from build123d import *

# Parameters (mm, degrees)
SKETCH1_R           = 6
BOSS_EXTRUDE1_DEPTH = 5
SKETCH2_R           = 5.262480872
BOSS_EXTRUDE2_DEPTH = 6
SKETCH3_R           = 0.5
CUT_EXTRUDE1_DEPTH  = 6
SKETCH4_R           = 6
BOSS_EXTRUDE3_DEPTH = 0.8
SKETCH5_R           = 4.819461856
BOSS_EXTRUDE4_DEPTH = 0.4
FILLET3_R           = 0.5
SKETCH6_R           = 4
CUT_EXTRUDE2_DEPTH  = 15.860686391


with BuildPart() as part:
    # Sketch1 → Boss-Extrude1 (new body)
    with BuildSketch(Plane(origin=(0, 0, 0), x_dir=(1, 0, 0), z_dir=(0, 1, 0))):
        with Locations(Location((0, 0, 0), (0, 0, 270))):
            Circle(SKETCH1_R)
    extrude(amount=BOSS_EXTRUDE1_DEPTH)

    # Sketch2 → Boss-Extrude2 (add)
    with BuildSketch(Plane(origin=(0, 5, 0), x_dir=(1, 0, 0), z_dir=(0, 1, 0))):
        with Locations(Location((0, 0, 0), (0, 0, 270))):
            Circle(SKETCH2_R)
    extrude(amount=BOSS_EXTRUDE2_DEPTH)

    # Sketch3 → Cut-Extrude1 (cut)
    with BuildSketch(Plane(origin=(0, 11, 0), x_dir=(1, 0, 0), z_dir=(0, 1, 0))):
        with Locations((-1.603876434, 5.012113856)):
            Circle(SKETCH3_R)
        with Locations((0.023451225, 5.262428619)):
            Circle(SKETCH3_R)
        with Locations((1.648483316, 4.997620202)):
            Circle(SKETCH3_R)
        with Locations((3.112150373, 4.2436099)):
            Circle(SKETCH3_R)
        with Locations((4.271178469, 3.074205493)):
            Circle(SKETCH3_R)
        with Locations((5.012113856, 1.603876434)):
            Circle(SKETCH3_R)
        with Locations((5.262428619, -0.023451225)):
            Circle(SKETCH3_R)
        with Locations((4.997620202, -1.648483316)):
            Circle(SKETCH3_R)
        with Locations((4.2436099, -3.112150373)):
            Circle(SKETCH3_R)
        with Locations((3.074205493, -4.271178469)):
            Circle(SKETCH3_R)
        with Locations((1.603876434, -5.012113856)):
            Circle(SKETCH3_R)
        with Locations((-0.023451225, -5.262428619)):
            Circle(SKETCH3_R)
        with Locations((-1.648483316, -4.997620202)):
            Circle(SKETCH3_R)
        with Locations((-3.112150373, -4.2436099)):
            Circle(SKETCH3_R)
        with Locations((-4.271178469, -3.074205493)):
            Circle(SKETCH3_R)
        with Locations((-5.012113856, -1.603876434)):
            Circle(SKETCH3_R)
        with Locations((-5.262428619, 0.023451225)):
            Circle(SKETCH3_R)
        with Locations((-4.997620202, 1.648483316)):
            Circle(SKETCH3_R)
        with Locations((-4.2436099, 3.112150373)):
            Circle(SKETCH3_R)
        with Locations((-3.074205493, 4.271178469)):
            Circle(SKETCH3_R)
    extrude(amount=-CUT_EXTRUDE1_DEPTH, mode=Mode.SUBTRACT)

    # Sketch4 → Boss-Extrude3 (add)
    with BuildSketch(Plane(origin=(0, 11, 0), x_dir=(1, 0, 0), z_dir=(0, 1, 0))):
        with Locations(Location((0, 0, 0), (0, 0, 270))):
            Circle(SKETCH4_R)
    extrude(amount=BOSS_EXTRUDE3_DEPTH)

    # Sketch5 → Boss-Extrude4 (add)
    with BuildSketch(Plane(origin=(0, 11.8, 0), x_dir=(1, 0, 0), z_dir=(0, 1, 0))):
        with Locations(Location((0, 0, 0), (0, 0, 270))):
            Circle(SKETCH5_R)
    extrude(amount=BOSS_EXTRUDE4_DEPTH)

    # Fillet3
    # the kernel refuses this fillet: 0.5 mm, written as the material it takes off along each edge
    with BuildSketch(Plane(origin=(0, 12.2, 0), x_dir=(0, 0, 1), z_dir=(-1, 0, 0))) as fillet3_piece_1:
        with BuildLine():
            CenterArc((4.329563907, -0.5), FILLET3_R, 11.536959033, 78.463040967)
            Line((4.329563907, 0), (4.329563907, 0.01))
            Line((4.329563907, 0.01), (4.819461856, 0.01))
            Line((4.819461856, 0.01), (4.829461856, 0))
            ThreePointArc((4.829461856, 0), (4.829461856, -0.2), (4.829259815, -0.398))
            Line((4.829259815, -0.398), (4.819461856, -0.4))
        make_face()
    revolve(axis=Axis((0, 12.2, 0), (0, 1, 0)), mode=Mode.SUBTRACT)

    # Sketch6 → Cut-Extrude2 (cut, through all)
    with BuildSketch(Plane(origin=(0, 12.2, 0), x_dir=(1, 0, 0), z_dir=(0, 1, 0))):
        with Locations(Location((0, 0, 0), (0, 0, 270))):
            Circle(SKETCH6_R)
    extrude(amount=-CUT_EXTRUDE2_DEPTH, mode=Mode.SUBTRACT)


solid = part.part
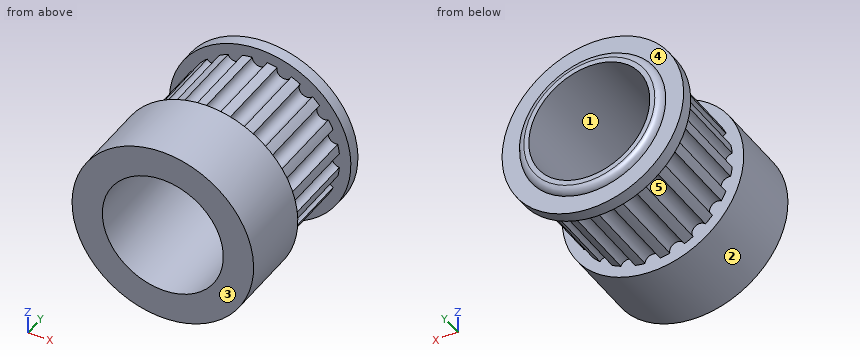
Read the model definition and answer for the solid it produces. Units are mm, in the model's axes. Face numbers are marked on the shaded views. A direction names the side the tool comes from. Coordinates: 2 decimals unless noted, no trailing zeros. Loops run counter-clockwise (first coordinate to the right, second up) from the corner with the lowest first, then second, coordinate; pieces in that order, holes last. Notation, with made-up numbers: (61.25, 27.5) -> (84.25, 27.5) arc R21 ccw to (84.25, 41.5) -> close; hole circle Ø10 at (64, -9). An arc over 180 degrees is marked (long way). Write item = value, one per line. Start each with the question number.
1) The part is cut by section B-B, the plane z = 0. Determine the outline of the cut face in (x, y), plus the area to 3 significant figures.
2) The part is cut by section A-A, the plane y = 3. Determine the outline of the cut face in (x, z), plus the area to 3 significant figures.
3) For the marked faces 4 and 5, determine the directions among +Z, -Z, +X, -X, +Y, -Y from which every point of the face is accessible in a straight line to the end or side of a thin tool.
4) Given P1, Ø3, axis at x = 2.5, y = 2.5, coming from the +Z side; P2, Ø2, axis at x = 1.5, y = 1.5, coming from the +Z side; P3, Ø7, axis at x = 0, z = 0, coming from the +Y side, each flat-ended and moving along its own axis, determine where each tip first touches the part or whether it passes through.
5) Find the intervals of material crossed by L1, parallel to Y at x = 3.25, z = 5; L2, parallel to X at y = 9.5, z = 0; L3, parallel to Z at x = -2, y = 6.25, in increasing order. Write a range as from..to.
6) The mould has two halves that part along X. Classify the marked faces 1, 2 and 3: pulls with the +X half, pulls with the -X half, needs draft (parallel to the pull), parting line crosses it, or undercut.
7) The part is cut by section C-C, the plane x = 0. Determine the outline of the cut face in (y, z), plus the area to 3 significant figures.
Result:
q1.outline = (-6, 0) -> (-4, 0) -> (-4, 12.2) -> (-4.33, 12.2) arc R0.5 ccw to (-4.82, 11.8) -> (-6, 11.8) -> (-6, 11) -> (-4.76, 11) -> (-4.76, 5) -> (-6, 5) -> close; (4, 0) -> (6, 0) -> (6, 5) -> (4.76, 5) -> (4.76, 11) -> (6, 11) -> (6, 11.8) -> (4.82, 11.8) arc R0.5 ccw to (4.33, 12.2) -> (4, 12.2) -> close
q1.area = 32.9 mm²
q2.outline = circle Ø12 at (0, 0); hole circle Ø8 at (0, 0)
q2.area = 62.8 mm²
q3.face_4 = +Y
q3.face_5 = none
q4.P1 = 5.92
q4.P2 = 5.98
q4.P3 = through
q5.L1 = 0..5, 11..11.8
q5.L2 = -4.76..-4, 4..4.76
q5.L3 = -4.71..-3.46, 3.46..4.64
q6.face_1 = undercut
q6.face_2 = parting line crosses it
q6.face_3 = needs draft
q7.outline = (0, -6) -> (5, -6) -> (5, -4.76) -> (11, -4.76) -> (11, -6) -> (11.8, -6) -> (11.8, -4.82) arc R0.5 ccw to (12.2, -4.33) -> (12.2, -4) -> (0, -4) -> close; (0, 4) -> (12.2, 4) -> (12.2, 4.33) arc R0.5 ccw to (11.8, 4.82) -> (11.8, 6) -> (11, 6) -> (11, 4.76) -> (5, 4.76) -> (5, 6) -> (0, 6) -> close
q7.area = 32.9 mm²
